The listing builds one solid part. Answer for the finished solid, in the listing's coordinates (mm). Give positions to 0.01 mm unless a question says otherwise; leave off trailing zeros. Loops run counter-clockwise (first coordinate to the right, second up) from the corner with the lowest first, then second, coordinate; pieces in that order, holes last. Notation, with made-up numbers: M 72.25,83 L 86.25,83 A21 ccw 86.25,92 Z; hole C 86,12.25 d8. An arc over 180 degrees is marked long. One line per item, written item: value. Start each with the question number.
Q1. A cutting plane is placed at A-A, the plane y = 75. Determine the outline of the cut face in (x, z), and give its area (3 significant figures).
Q2. Consider L1, parallel to Z at x = -4, y = 75; L2, parallel to Y at x = -0.75, z = -2.5. Determine where each line is inside the solid, lowest interval first.
Q3. A cutting plane is placed at B-B, the plane z = 0. Determine the outline of the cut face in (x, y), and give its area (3 significant figures).
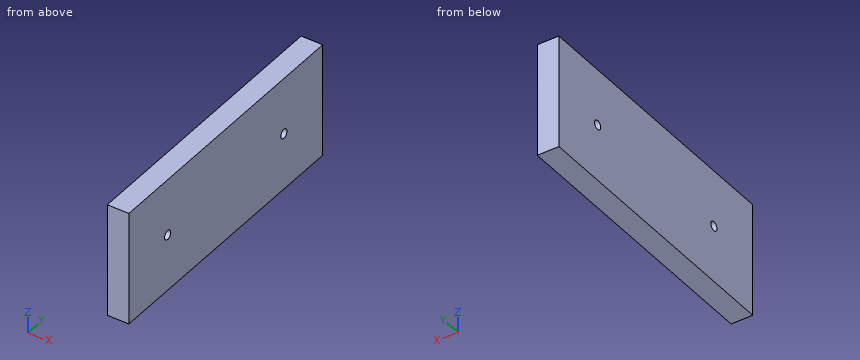
Autodesk Inventor part; units mm, degrees
ref_plane "YZ Plane" through (0, 0, 0) normal (1, 0, 0) x (0, 1, 0)
ref_plane "XZ Plane" through (0, 0, 0) normal (0, 1, 0) x (-1, 0, 0)
ref_plane "XY Plane" through (0, 0, 0) normal (0, 0, 1) x (1, 0, 0)
sketch "Sketch1" plane through (0, 0, 0) normal (1, 0, 0) x (0, 1, 0)
  line L0 (125, 50) -> (-125, 50)
  line L1 (-125, 50) -> (-125, -50)
  line L2 (-125, -50) -> (125, -50)
  line L3 (125, -50) -> (125, 50)
  line L4 (125, 50) -> (-125, -50) construction
  line L5 (-125, 50) -> (125, -50) construction
  line L6 (125, 0) -> (75, 0)
  line L7 (-125, 0) -> (-75, 0)
  circle A0 centre (-75, 0) radius 4
  circle A1 centre (75, 0) radius 4
  point P0 (0, 0)
  dimension "d0" = 250
  dimension "d1" = 100
  dimension "d2" = 50
  dimension "d3" = 50
  dimension "d4" = 8
  dimension "d5" = 8
extrude "Extrusion1" add sketch "Sketch1" along normal mid plane 19
properties part number "H"
Answer block:
1. outline: M -9.5,-50 L 9.5,-50 L 9.5,-4 L -9.5,-4 Z; M -9.5,4 L 9.5,4 L 9.5,50 L -9.5,50 Z
1. area: 1,750 mm^2
2. L1: -50 to -4, 4 to 50
2. L2: -125 to -78.12, -71.88 to 71.88, 78.12 to 125
3. outline: M -9.5,-125 L 9.5,-125 L 9.5,-79 L -9.5,-79 Z; M -9.5,-71 L 9.5,-71 L 9.5,71 L -9.5,71 Z; M -9.5,79 L 9.5,79 L 9.5,125 L -9.5,125 Z
3. area: 4,450 mm^2
